Build history of the part. All positions in model axes, mm. Face numbers are marked on the shaded views. A direction names the side the tool comes from. Give positions to 0.01 mm unless a question says otherwise; leave off trailing zeros. Loops run counter-clockwise (first coordinate to the right, second up) from the corner with the lowest first, then second, coordinate; pieces in that order, holes last. Notation, with made-up numbers: (-27.5, -14) -> (14.5, -14) arc R9 ccw to (14.5, 2) -> close; hole circle Ø8 at (72, -28). An arc over 180 degrees is marked (long way). Answer as a JSON object with one key per item and string values. Group by question number.
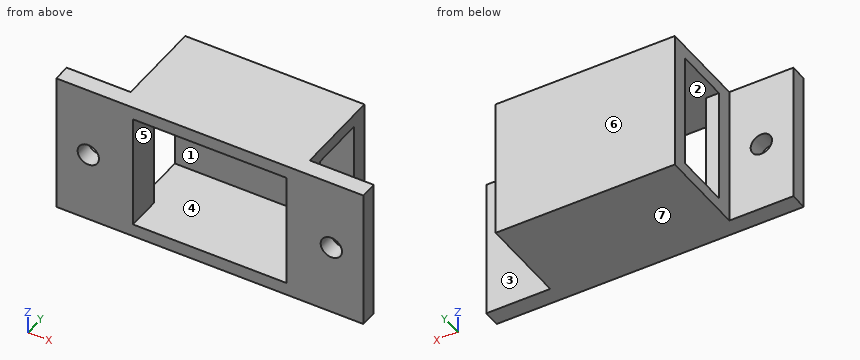
from build123d import *

# Parameters (mm, degrees)
SKETCH_1_W          = 42
SKETCH_1_H          = 33
EXTRUDE_1_DEPTH     = 25
SKETCH_2_W          = 72
SKETCH_2_H          = 33
EXTRUDE_2_DEPTH     = 4
SKETCH_3_W          = 36
SKETCH_3_H          = 27
CUT_EXTRUDE_1_DEPTH = 21
SKETCH_4_W          = 27
SKETCH_4_H          = 13
CUT_EXTRUDE_2_DEPTH = 58
SKETCH_5_R          = 2.5
CUT_EXTRUDE_3_DEPTH = 26


with BuildPart() as part:
    # 草圖1 → 填料-伸長1 (new body)
    with BuildSketch(Plane(origin=(0, 0, 0), x_dir=(1, 0, 0), z_dir=(0, 1, 0))):
        Rectangle(SKETCH_1_W, SKETCH_1_H)
    extrude(amount=EXTRUDE_1_DEPTH)

    # 草圖2 → 填料-伸長2 (add)
    with BuildSketch(Plane(origin=(0, 0, 0), x_dir=(1, 0, 0), z_dir=(0, 1, 0))):
        Rectangle(SKETCH_2_W, SKETCH_2_H)
    extrude(amount=EXTRUDE_2_DEPTH)

    # 草圖3 → 除料-伸長1 (cut)
    with BuildSketch(Plane.XZ):
        Rectangle(SKETCH_3_W, SKETCH_3_H)
    extrude(amount=-CUT_EXTRUDE_1_DEPTH, mode=Mode.SUBTRACT)

    # 草圖4 → 除料-伸長2 (cut, through all)
    with BuildSketch(Plane.ZY.offset(21)):
        with Locations((0, 14.5)):
            Rectangle(SKETCH_4_W, SKETCH_4_H)
    extrude(amount=-CUT_EXTRUDE_2_DEPTH, mode=Mode.SUBTRACT)

    # 草圖5 → 除料-伸長3 (cut, through all)
    with BuildSketch(Plane.XZ):
        with Locations((28.5, 0)):
            Circle(SKETCH_5_R)
        with Locations((-28.5, 0)):
            Circle(SKETCH_5_R)
    extrude(amount=-CUT_EXTRUDE_3_DEPTH, mode=Mode.SUBTRACT)


solid = part.part
(1) Pin check, flat tips, straight feed: pin 1 (10.5 mm diameter, centred on y = 18.5, z = 6, fed in from -X); pin 2 (8 mm diameter, centred on x = 6, z = 6, fed in from -Y); pin 3 (3 mm diameter, centred on x = 28.5, z = 0, fed in from +Y). Stop position of each tip, or through.
(2) Pull direction Z, two halves, no side cores. Call the marked faces 4, 5, 6 and 7: pulls with the +Z half, pulls with the -Z half, needs draft (parallel to the pull), parting line crosses it, or undercut.
(3) Saw through at D-D on y = 5. List the corners of the cut face in (x, z), plus the area to 3 significant figures.
(4) Saw through at A-A on y = 17.25. List the corners of the cut face in (x, z), plus the area to 3 significant figures.
(5) Saw through at B-B on x = 28.5. List the corners of the cut face in (y, z), plus the area to 3 significant figures.
(6) Probe line 1 along Z through (x, y) = (-14, 15.5); line 2 along Z through (x, y) = (-28.5, 1.15); line 3 along Y through (x, z) = (18.5, 4.5). List the from-to ranges inside material, lowest first. Write a range as [from, to].
(7) Saw through at C-C on z = 9. List the corners of the cut face in (x, y).
(8) 3-axis set-ups, long thin cutter, end or side, ignore diameter. For the marked faces 1, 2 and 3: which of +Z, -Z, +X, -X, +Y, -Y reach the whole face in a straight line?
Calculated:
{
 "1": {"pin 1": "stops at x = -21", "pin 2": "stops at y = 21", "pin 3": "passes through"},
 "2": {"face 4": "undercut", "face 5": "undercut", "face 6": "needs draft", "face 7": "pulls with the -Z half"},
 "3": {"outline": "(-21, -16.5) -> (21, -16.5) -> (21, 16.5) -> (-21, 16.5) -> close; hole (-18, -13.5) -> (18, -13.5) -> (18, 13.5) -> (-18, 13.5) -> close", "area": "414 mm^2"},
 "4": {"outline": "(-21, -16.5) -> (21, -16.5) -> (21, -13.5) -> (-21, -13.5) -> close; (-21, 13.5) -> (21, 13.5) -> (21, 16.5) -> (-21, 16.5) -> close", "area": "252 mm^2"},
 "5": {"outline": "(0, -16.5) -> (4, -16.5) -> (4, -2.5) -> (0, -2.5) -> close; (0, 2.5) -> (4, 2.5) -> (4, 16.5) -> (0, 16.5) -> close", "area": "112 mm^2"},
 "6": {"line 1": "z = [-16.5, -13.5], [13.5, 16.5]", "line 2": "z = [-16.5, -2.5], [2.5, 16.5]", "line 3": "y = [0, 8], [21, 25]"},
 "7": {"outline": "(-36, 0) -> (-18, 0) -> (-18, 8) -> (-21, 8) -> (-21, 4) -> (-36, 4) -> close; (-21, 21) -> (21, 21) -> (21, 25) -> (-21, 25) -> close; (18, 0) -> (36, 0) -> (36, 4) -> (21, 4) -> (21, 8) -> (18, 8) -> close"},
 "8": {"face 1": "+X, -X", "face 2": "none", "face 3": "+Z, -Z, +X, +Y"}
}
